Build history of the part. All positions in model axes, mm. A direction names the side the tool comes from. Coordinates: 2 decimals unless noted, no trailing zeros. Loops run counter-clockwise (first coordinate to the right, second up) from the corner with the lowest first, then second, coordinate; pieces in that order, holes last.
(1) Tool access for faces 4 (the face through (12, 27, -28)), 5 (the face through (10, 10, -2)): list every direction of +Z, -Z, +X, -X, +Y, -Y with a clear straight run to the whole face (end or side of a thin tool).
(2) Slice it at C-C (z = -30). Give the cut face in (x, y).
(3) Slice it at D-D (y = 13.5). Give the cut face in (x, z).
(4) Flat gauge pins, fed straight in: P1, Ø1, axis at y = 23, z = -44, coming from the +X side; P2, Ø12, axis at x = 7.5, y = 5, coming from the -Z side; P3, Ø5, axis at x = 12.5, z = -10, coming from the -Y side. Where does each tip first touch, or does it go through?
(5) Wall check: L1, parallel to X at y = 26.25, z = -20; L2, parallel to Z at x = 19.5, y = 5.75; L3, parallel to Y at x = 21, z = -0.4. Give the ranges that are in metal, low to high.
(6) Two-plate mould, pull along X, no slides. Class faces 1 (the face through (10, 25, -29)), 2 (the face through (19.5, 13.57, -0.99)), 3 (the face through (0, 26, -20)): pulls with the +X half, pulls with the -X half, needs draft (parallel to the pull), parting line crosses it, or undercut.
(7) Slice it at A-A (y = 5). Give the cut face in (x, z), and give its area (3 significant figures).
(8) Slice it at B-B (x = 21). Give the cut face in (y, z), and give its area (3 significant figures).
from build123d import *

# Parameters (mm, degrees)
BOSS_EXTRUDE1_DEPTH = 25
SKETCH2_R           = 1.5
SKETCH2_R_2         = 3.5
CUT_EXTRUDE1_DEPTH  = 25
SKETCH3_R           = 1.5
CUT_EXTRUDE2_DEPTH  = 25


with BuildPart() as part:
    # Sketch1 → Boss-Extrude1 (new body)
    with BuildSketch(Plane(origin=(0, 0, 0), x_dir=(0, 0, -1), z_dir=(1, 0, 0))):
        Polygon((0, 0), (0, 27), (56, 27), (56, 25), (2, 25), (2, 0), align=None)
    extrude(amount=BOSS_EXTRUDE1_DEPTH)

    # Sketch2 → Cut-Extrude1 (cut)
    with BuildSketch(Plane.XY):
        with Locations((4, 13.5)):
            Circle(SKETCH2_R)
        with Locations((12.5, 13.5)):
            Circle(SKETCH2_R_2)
        with Locations((12.5, 22)):
            Circle(SKETCH2_R)
        with Locations((21, 13.5)):
            Circle(SKETCH2_R)
        with Locations((12.5, 5)):
            Circle(SKETCH2_R)
    extrude(amount=-CUT_EXTRUDE1_DEPTH, mode=Mode.SUBTRACT)

    # Sketch3 → Cut-Extrude2 (cut)
    with BuildSketch(Plane(origin=(0, 27, 0), x_dir=(1, 0, 0), z_dir=(0, 1, 0))):
        with Locations(Location((12.5, 10, 0), (0, 0, 270))):
            Circle(SKETCH3_R)
        with Locations(Location((12.5, 20, 0), (0, 0, 270))):
            Circle(SKETCH3_R)
        with Locations(Location((12.5, 30, 0), (0, 0, 270))):
            Circle(SKETCH3_R)
        with Locations(Location((12.5, 40, 0), (0, 0, 270))):
            Circle(SKETCH3_R)
        with Locations(Location((12.5, 50, 0), (0, 0, 270))):
            Circle(SKETCH3_R)
    extrude(amount=-CUT_EXTRUDE2_DEPTH, mode=Mode.SUBTRACT)


solid = part.part
Response values:
1. face 4: +Z, -Z, +X, -X, +Y
1. face 5: -Z, +X, -X, -Y
2. outline: (0, 25) - (11, 25) - (11, 27) - (0, 27) - close; (14, 25) - (25, 25) - (25, 27) - (14, 27) - close
3. outline: (0, -2) - (2.5, -2) - (2.5, 0) - (0, 0) - close; (5.5, -2) - (9, -2) - (9, 0) - (5.5, 0) - close; (16, -2) - (19.5, -2) - (19.5, 0) - (16, 0) - close; (22.5, -2) - (25, -2) - (25, 0) - (22.5, 0) - close
4. P1: passes through
4. P2: stops at z = -2
4. P3: stops at y = 25
5. L1: x = 0 to 11, 14 to 25
5. L2: z = -2 to 0
5. L3: y = 0 to 12, 15 to 27
6. face 1: needs draft
6. face 2: undercut
6. face 3: pulls with the -X half
7. outline: (0, -2) - (11, -2) - (11, 0) - (0, 0) - close; (14, -2) - (25, -2) - (25, 0) - (14, 0) - close
7. area: 44.0 mm2
8. outline: (0, -2) - (12, -2) - (12, 0) - (0, 0) - close; (15, -2) - (25, -2) - (25, -56) - (27, -56) - (27, 0) - (15, 0) - close
8. area: 156 mm2
